Check sheet for the modelled part. Datum: model origin and axes. Units: mm. A direction names the side the tool comes from. Coordinates: 2 decimals unless noted, no trailing zeros. Write each loop counter-clockwise with the first axis right and the second up, starting at its lowest first coordinate (ties: lowest second). Pieces come first, ordered by that corner, then holes. Notation, with made-up numbers: M 68.25,-9 L 87.25,-9 A24 ccw 87.25,8 Z; hole C 17,-40 d4. An arc over 180 degrees is marked long. Answer as CSV lines item,"result". Start each with the question number.
1) Section check C-C (x = 39.5). Record the cut outline in (y, z).
2) Section check D-D (x = 6). Record the cut outline in (y, z).
3) Draft check along Y on faces 3 (the flat face through (75, -11, 24)), 4 (the cylindrical face through (36.989, -7.509, 23.846)), 5 (the cylindrical face through (47.378, 32.825, 17.073)). Enter one of: +Y half, -Y half, draft (parallel to the pull), parting line (faces both ways), or undercut.
4) Section check A-A (z = 0). Record the cut outline in (x, y), and give its area (3 significant figures).
5) Material ranges on L1, parallel to Y at x = 50, z = 0; L2, parallel to Y at x = 10.5, z = 14; L3, parallel to Z at x = 30.5, y = 11.5, recorded low to high. Write a range as [from, to].
6) Go/stop test with flat-tipped pins: pin 1 Ø10 at (y, z) = (-1.5, -20) entering from -X; pin 2 Ø5 at (x, z) = (32, 5) entering from -Y; pin 3 Ø1.5 at (x, y) = (33.5, 26.5) entering from +Z. Record where each tip stops, or that it passes through.
7) Access from +Z, -Z, +X, -X, +Y, -Y to the whole of each face (thin tool, end or side, straight path). Record for faces 1 (the cylindrical face through (10.633, 37.096, -8.238)), 2 (the flat face through (20, 36.4, 8.3)).
from build123d import *

# Parameters (mm, degrees)
CHAMFER_1_SIZE = 1


with BuildPart() as part:
    # 草图1 → 旋转1 (revolve)
    with BuildSketch(Plane.XY, mode=Mode.PRIVATE) as revolve_1_sk:
        Polygon((0, 25), (0, 38), (20, 38), (20, 37), (75, 37), (75, 25), align=None)
    revolve(revolve_1_sk.sketch.rotate(Axis((0, 0, 0), (1, 0, 0)), 90), axis=Axis((0, 0, 0), (1, 0, 0)))

    # 倒角1
    chamfer_1_edges = [part.edges().sort_by_distance(p)[0] for p in [
        (75, 0, -25),
        (75, 0, -37),
        (0, 0, -38),
        (0, 0, -25),
    ]]
    chamfer(chamfer_1_edges, length=CHAMFER_1_SIZE)


solid = part.part
Results found:
1,outline,"C 0,0 d74; hole C 0,0 d50"
2,outline,"C 0,0 d76; hole C 0,0 d50"
3,face 3,"draft"
3,face 4,"undercut"
3,face 5,"parting line"
4,outline,"M 0,-37 L 1,-38 L 20,-38 L 20,-37 L 74,-37 L 75,-36 L 75,-26 L 74,-25 L 1,-25 L 0,-26 Z; M 0,26 L 1,25 L 74,25 L 75,26 L 75,36 L 74,37 L 20,37 L 20,38 L 1,38 L 0,37 Z"
4,area,"1,840 mm2"
5,L1,"y = [-37, -25], [25, 37]"
5,L2,"y = [-35.33, -20.71], [20.71, 35.33]"
5,L3,"z = [-35.17, -22.2], [22.2, 35.17]"
6,pin 1,"stops at x = 0.94"
6,pin 2,"stops at y = -36.92"
6,pin 3,"stops at z = 26.57"
7,face 1,"+X, -X"
7,face 2,"+X"
